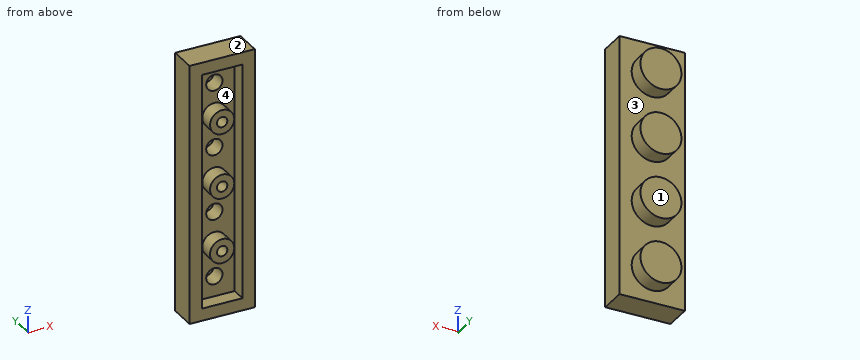
Autodesk Inventor part; units mm, degrees
ref_plane "YZ Plane" through (0, 0, 0) normal (1, 0, 0) x (0, 1, 0)
ref_plane "XZ Plane" through (0, 0, 0) normal (0, 1, 0) x (-1, 0, 0)
ref_plane "XY Plane" through (0, 0, 0) normal (0, 0, 1) x (1, 0, 0)
sketch "Sketch1" plane through (0, 0, 0) normal (0, 1, 0) x (-1, 0, 0)
  line L0 (0, 0) -> (7.7978, 0)
  line L1 (7.7978, 0) -> (7.7978, -31.1912)
  line L2 (7.7978, -31.1912) -> (0, -31.1912)
  line L3 (0, -31.1912) -> (0, 0)
  dimension "d0" = 7.7978
  dimension "d1" = 31.1912
extrude "Extrusion1" add sketch "Sketch1" along normal blind 3.236
sketch "Sketch2" plane through (0, 3.236, 0) normal (0, 1, 0) x (1, 0, 0)
  line L0 (0, 0) -> (-3.8989, 0) construction
  line L1 (-3.8989, 0) -> (-3.8989, 3.8989) construction
  line L2 (-3.8989, 3.8989) -> (0, 3.8989) construction
  line L3 (0, 3.8989) -> (0, 0) construction
  circle A0 centre (-3.8989, 3.8989) radius 2.4498
  dimension "d4" = 3.8989
  dimension "d5" = 3.8989
  dimension "d6" = 4.8997
extrude "Extrusion2" add sketch "Sketch2" along normal blind 1.9837
pattern_linear "Rectangular Pattern1" count 4 spacing 7.7978 along (0, 0, -1) of "Extrusion2"
shell "Shell1" thickness 1.4732 removed faces 1 at (-2.5993, 0, -10.3971)
sketch "Sketch3" plane through (-6.3246, 1.7628, -1.4732) normal (0, -1, 0) x (1, 0, 0)
  circle A0 centre (2.4257, -2.4257) radius 2.4498 construction
  circle A1 centre (2.4257, -10.2235) radius 2.4498 construction
  line L0 (2.4257, -2.4257) -> (2.4257, -10.2235) construction
  circle A2 centre (2.4257, -6.3246) radius 0.6198
  circle A3 centre (2.4257, -6.3246) radius 1.4491
  point P0 (6.3246, 1.4732)
  dimension "d13" = 1.2395
extrude "Extrusion3" add sketch "Sketch3" along normal up to surface (1.7628 mm away)
pattern_linear "Rectangular Pattern2" count 3 spacing 7.7978 along (0, 0, -1) of "Extrusion3"
properties part number "1x4 short black pegged" material "ABS Plastic"
Model file for the job. Use its own axes, mm. Face numbers are marked on the shaded views. Coordinates: 2 decimals unless noted, no trailing zeros. Order: outer loops, then holes, each group sorted by start corner. A loop starts at its lowest first (then second) coordinate and runs counter-clockwise, first axis right, second up. Notation, with made-up numbers: (-19, 62.25) -> (-12, 62.25) arc R29 ccw to (-12, 89.25) -> close; hole circle Ø4 at (83, 87). An arc over 180 degrees is marked (long way). Return JSON: item names as keys, results as strings. Group by question number.
Item 1: Saw through at A-A on y = 1.35. Write the cut outline in (x, z), then the cut area to 3 significant figures.
Item 2: Saw through at D-D on x = -0.5. Write the cut outline in (y, z).
Item 3: Flat gauge pins, fed straight in: P1, Ø1.6, axis at x = -4, z = -11.5, coming from the -Y side; P2, Ø1.1, axis at x = -3.9, z = -23.39, coming from the +Y side; P3, Ø1.6, axis at x = -3.9, z = -27.29, coming from the -Y side. Where does each tip first touch, or does it go through?
Item 4: Saw through at C-C on y = 4.75. Write the cut outline in (x, z).
Item 5: Pull direction Z, two halves, no side cores. Call the marked faces 1, 2, 3 and 4: pulls with the +Z half, pulls with the -Z half, needs draft (parallel to the pull), parting line crosses it, or undercut.
Item 6: Saw through at B-B on z = -24.5. Write the cut outline in (x, y).
Item 7: Wall check: line 1 along X through (y, z) = (1.35, -10.5); line 2 along Z through (x, y) = (-2.25, 0.25); line 3 along Z through (x, y) = (-4.25, 4.7). Give the ranges that are in metal, low to high. Write a range as [from, to].
Values found:
{
 "1": {"outline": "(-7.8, -31.19) -> (0, -31.19) -> (0, 0) -> (-7.8, 0) -> close; circle Ø2.9 at (-3.9, -23.39); circle Ø2.9 at (-3.9, -15.6); circle Ø2.9 at (-3.9, -7.8); hole (-6.32, -29.72) -> (-1.47, -29.72) -> (-1.47, -1.47) -> (-6.32, -1.47) -> close; hole circle Ø1.24 at (-3.9, -23.39); hole circle Ø1.24 at (-3.9, -15.6); hole circle Ø1.24 at (-3.9, -7.8)", "area": "122 mm2"},
 "2": {"outline": "(0, -31.19) -> (3.24, -31.19) -> (3.24, 0) -> (0, 0) -> close"},
 "3": {"P1": "stops at y = 1.76", "P2": "stops at y = 3.24", "P3": "stops at y = 3.75"},
 "4": {"outline": "circle Ø4.9 at (-3.9, -27.29); circle Ø4.9 at (-3.9, -19.49); circle Ø4.9 at (-3.9, -11.7); circle Ø4.9 at (-3.9, -3.9)"},
 "5": {"face 1": "needs draft", "face 2": "pulls with the +Z half", "face 3": "undercut", "face 4": "undercut"},
 "6": {"outline": "(-7.8, 0) -> (-6.32, 0) -> (-6.32, 1.76) -> (-4.83, 1.76) -> (-4.83, 0) -> (-2.96, 0) -> (-2.96, 1.76) -> (-1.47, 1.76) -> (-1.47, 0) -> (0, 0) -> (0, 3.24) -> (-7.8, 3.24) -> close"},
 "7": {"line 1": "x = [-7.8, -6.32], [-1.47, 0]", "line 2": "z = [-31.19, -29.72], [-1.47, 0]", "line 3": "z = [-29.72, -24.87], [-21.92, -17.07], [-14.12, -9.27], [-6.32, -1.47]"}
}
